Source: CAD feature listing. Evaluate the final solid. Frame: model axes, mm. Give positions to 0.01 mm unless a question says otherwise; leave off trailing zeros. Loops run counter-clockwise (first coordinate to the right, second up) from the corner with the lowest first, then second, coordinate; pieces in that order, holes last. Notation, with made-up numbers: M 47.25,-2.75 L 84.25,-2.75 A28 cw 84.25,30.25 Z; hole C 61,27 d8. An arc over 180 degrees is marked long. Answer in a Markdown table with one row per item.
```python
from build123d import *

# Parameters (mm, degrees)
SKETCH1_W                = 304.8
SKETCH1_H                = 241.3
BOSS_EXTRUDE4_DEPTH      = 6.35
SKETCH3_W                = 6.35
SKETCH3_H                = 25.470512821
SKETCH3_H_2              = 25.4
SMALL_TEETH_CUT_DEPTH    = 7.62
BIG_TEETH_CUT_DEPTH      = 360.242006362
BIG_TEETH_CUT_DEPTH_BACK = 360.242006362
BIG_TEETH_W              = 25.4
BIG_TEETH_H              = 25.4
SKETCH4_W                = 152.4
SKETCH4_H                = 6.35
CUT_EXTRUDE1_DEPTH       = 360.242006362
SKETCH5_W                = 18.365609198
SKETCH5_H                = 25.315792254
CUT_EXTRUDE2_DEPTH       = 360.242006362
SKETCH6_W                = 152.4
SKETCH6_H                = 6.35
CUT_EXTRUDE3_DEPTH       = 360.242006362


with BuildPart() as part:
    # Sketch1 → Boss-Extrude4 (new body)
    with BuildSketch(Plane(origin=(0, 0, 0), x_dir=(0, 0, -1), z_dir=(1, 0, 0))):
        with Locations((-173.678767452, 29.972488533)):
            Rectangle(SKETCH1_W, SKETCH1_H)
    extrude(amount=BOSS_EXTRUDE4_DEPTH)

    # Sketch3 → Small_teeth_cut (cut)
    with BuildSketch(Plane.ZY):
        with Locations((24.453767452, -77.942255057)):
            Rectangle(SKETCH3_W, SKETCH3_H)
        with Locations((24.453767452, -27.106998646)):
            Rectangle(SKETCH3_W, SKETCH3_H_2)
        with Locations((24.453767452, 23.693001354)):
            Rectangle(SKETCH3_W, SKETCH3_H_2)
        with Locations((24.453767452, 74.493001354)):
            Rectangle(SKETCH3_W, SKETCH3_H_2)
        with Locations((24.453767452, 125.293001354)):
            Rectangle(SKETCH3_W, SKETCH3_H_2)
    extrude(amount=-SMALL_TEETH_CUT_DEPTH, mode=Mode.SUBTRACT)

    # big teeth → Big_teeth_cut (cut, two sides: drawn at the far end of the back side and taken through both)
    with BuildSketch(Plane(origin=(6.35, 0, 0), x_dir=(0, 0, -1), z_dir=(1, 0, 0)).offset(-BIG_TEETH_CUT_DEPTH_BACK)):
        with Locations((-313.378767452, -77.977511467)):
            Rectangle(BIG_TEETH_W, BIG_TEETH_H)
        with Locations((-313.378767452, -27.177511467)):
            Rectangle(BIG_TEETH_W, BIG_TEETH_H)
        with Locations((-313.378767452, 23.622488533)):
            Rectangle(BIG_TEETH_W, BIG_TEETH_H)
        with Locations((-313.378767452, 74.422488533)):
            Rectangle(BIG_TEETH_W, BIG_TEETH_H)
        with Locations((-313.378767452, 125.222488533)):
            Rectangle(BIG_TEETH_W, BIG_TEETH_H)
    extrude(amount=BIG_TEETH_CUT_DEPTH + BIG_TEETH_CUT_DEPTH_BACK, mode=Mode.SUBTRACT)

    # Sketch4 → Cut-Extrude1 (cut, through all)
    with BuildSketch(Plane(origin=(6.35, 0, 0), x_dir=(0, 0, -1), z_dir=(1, 0, 0))):
        with Locations((-173.678767452, 147.447488533)):
            Rectangle(SKETCH4_W, SKETCH4_H)
    extrude(amount=-CUT_EXTRUDE1_DEPTH, mode=Mode.SUBTRACT)

    # Sketch5 → Cut-Extrude2 (cut, through all)
    with BuildSketch(Plane.ZY):
        with Locations((251.315206335, -78.01961534)):
            Rectangle(SKETCH5_W, SKETCH5_H)
    extrude(amount=-CUT_EXTRUDE2_DEPTH, mode=Mode.SUBTRACT)

    # Sketch6 → Cut-Extrude3 (cut, through all)
    with BuildSketch(Plane.ZY):
        with Locations((173.678767452, -44.322511467)):
            Rectangle(SKETCH6_W, SKETCH6_H)
    extrude(amount=-CUT_EXTRUDE3_DEPTH, mode=Mode.SUBTRACT)


solid = part.part
```
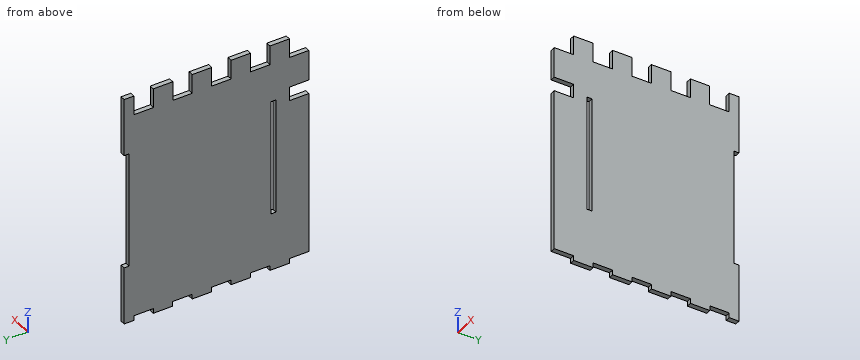
Q1. Section query A-A (z = 226). Output: boundary loops of the cut face in (x, y).
Values follow:
| item | result |
|---|---|
| outline | M 0,-90.68 L 6.35,-90.68 L 6.35,-47.5 L 0,-47.5 Z; M 0,-41.15 L 6.35,-41.15 L 6.35,144.27 L 0,144.27 Z |
Q2. Contact query for flat-ended pins moving along their axis: pin 1 Ø3 at (x, y) = (2, -31.5) entering from +Z; pin 2 Ø1.9 at (x, z) = (3.5, 315) entering from -Y; pin 3 Ø3 at (x, z) = (4.5, 24.5) entering from -Y. Output: stop coordinate, or through.
Values follow:
| item | result |
|---|---|
| pin 1 | z = 300.68 |
| pin 2 | y = -65.28 |
| pin 3 | y = -65.21 |
Q3. Ray query, probe 1 along Y at (x, z) = (2.25, 309); probe 2 along Y at (x, z) = (2, 196); probe 3 along Y at (x, z) = (5.25, 242.5). Return the intervals inside material, ascending. Write a range as from..to.
Values follow:
| item | result |
|---|---|
| probe 1 | -65.28..-39.88, -14.48..10.92, 36.32..61.72, 87.12..112.52, 137.92..150.62 |
| probe 2 | -90.68..-47.5, -41.15..144.27 |
| probe 3 | -65.36..-47.5, -41.15..144.27 |
Q4. Section query B-B (y = 70). Output: boundary loops of the cut face in (x, z), plus the area to 3 significant figures.
Values follow:
| item | result |
|---|---|
| outline | M 0,27.63 L 6.35,27.63 L 6.35,300.68 L 0,300.68 Z |
| area | 1,730 mm^2 |
